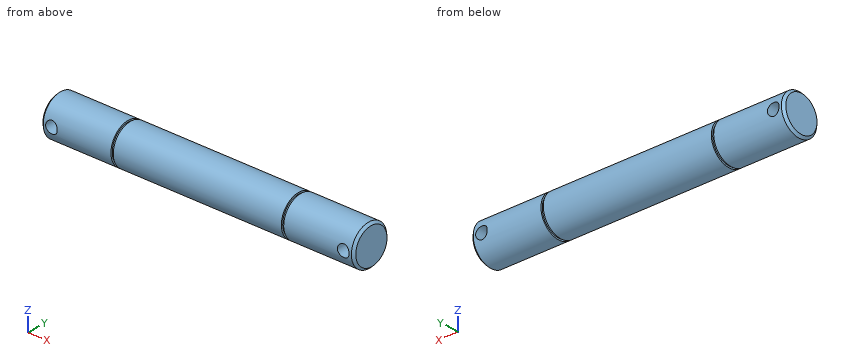
from build123d import *

# Parameters (mm, degrees)
SKETCH1_R               = 8.5
BOSS_EXTRUDE1_DEPTH     = 134
CHAMFER1_SIZE           = 1
SKETCH2_R               = 2.5
CUT_EXTRUDE1_DEPTH      = 9.5
CUT_EXTRUDE1_DEPTH_BACK = 9.5
SKETCH3_R               = 8.5
SKETCH3_R_2             = 7.85
CUT_EXTRUDE2_DEPTH      = 1


with BuildPart() as part:
    # Sketch1 → Boss-Extrude1 (new body)
    with BuildSketch(Plane(origin=(0, 0, 0), x_dir=(0, 0, -1), z_dir=(1, 0, 0))):
        Circle(SKETCH1_R)
    extrude(amount=BOSS_EXTRUDE1_DEPTH)

    # Chamfer1
    chamfer1_edges = [part.edges().sort_by_distance(p)[0] for p in [
        (0, 0, 8.5),
        (134, 0, 8.5),
    ]]
    chamfer(chamfer1_edges, length=CHAMFER1_SIZE)

    # Sketch2 → Cut-Extrude1 (cut, two sides)
    with BuildSketch(Plane(origin=(0, 0, 0), x_dir=(1, 0, 0), z_dir=(0, 1, 0))) as cut_extrude1_sk:
        with Locations((4.5, 0)):
            Circle(SKETCH2_R)
        with Locations((129.5, 0)):
            Circle(SKETCH2_R)
    extrude(amount=CUT_EXTRUDE1_DEPTH, mode=Mode.SUBTRACT)
    extrude(cut_extrude1_sk.sketch, amount=-CUT_EXTRUDE1_DEPTH_BACK, mode=Mode.SUBTRACT)

    # Sketch3 → Cut-Extrude2 (cut)
    with BuildSketch(Plane(origin=(104, 0, 0), x_dir=(0, 0, -1), z_dir=(1, 0, 0))):
        Circle(SKETCH3_R)
        Circle(SKETCH3_R_2, mode=Mode.SUBTRACT)
    cut_extrude2 = extrude(amount=-CUT_EXTRUDE2_DEPTH, mode=Mode.SUBTRACT)

    # Mirror1: Cut-Extrude2 across plane
    add(cut_extrude2.mirror(Plane(origin=(67, 0, 0), x_dir=(0, 0, 1), z_dir=(1, 0, 0))), mode=Mode.SUBTRACT)


solid = part.part
Could you check a few things on this model? Use its own coordinates, in mm. Give positions to 0.01 mm unless a question says otherwise; leave off trailing zeros. Order: outer loops, then holes, each group sorted by start corner. A loop starts at its lowest first (then second) coordinate and runs counter-clockwise, first axis right, second up. Notation, with made-up numbers: (73, 86.25) -> (90, 86.25) arc R12 cw to (90, 102.25) -> close; hole circle Ø5 at (-30.5, 75.25). An arc over 180 degrees is marked (long way). Answer in a Markdown table with one row per item. Add a question column.
Item 1: Imagine slicing it at A-A (z = 0). Count the separate pieces of the cut face and the enclosed holes in it, and give its area (3 significant figures).
Item 2: Please list where these lines run through material, in increasing order: probe 1 along X at (y, z) = (2.75, 0); probe 2 along X at (y, z) = (5.5, 0.5); probe 3 along Z at (x, y) = (128.5, -4.25).
Item 3: Imagine slicing it at B-B (x = 85.5). List the corners of the cut face in (y, z) for me.
Item 4: Imagine slicing it at D-D (x = 4.5). List the corners of the cut face in (y, z) for me, and give its area (3 significant figures).
Item 5: I'm going to push flat-ended pins straight in: P1, Ø1, axis at x = 51.5, z = 2, coming from the -Y side; P2, Ø4, axis at x = 37.5, z = 5, coming from the -Y side; P3, Ø2, axis at x = 112, z = 3.5, coming from the +Y side; P4, Ø3, axis at x = 4.5, z = 0, coming from the +Y side. Where does each tip first touch, or does it pass through?
Result:
| question | item | result |
|---|---|---|
| 1 | separate pieces | 3 |
| 1 | enclosed holes | 0 |
| 1 | area | 2,100 mm2 |
| 2 | probe 1 | 0 to 2, 7 to 127, 132 to 134 |
| 2 | probe 2 | 0 to 2.05, 6.95 to 127.05, 131.95 to 134 |
| 2 | probe 3 | -7.36 to -2.29, 2.29 to 7.36 |
| 3 | outline | circle Ø17 at (0, 0) |
| 4 | outline | (-8.12, -2.5) arc R8.5 ccw to (8.12, -2.5) -> close; (-8.12, 2.5) -> (8.12, 2.5) arc R8.5 ccw to start |
| 4 | area | 143 mm2 |
| 5 | P1 | y = -8.37 |
| 5 | P2 | y = -7.95 |
| 5 | P3 | y = 8.12 |
| 5 | P4 | through |
